For this review, take the finished solid that the model builds, in its own axes (mm). Face numbers are marked on the shaded views. A direction names the side the tool comes from. Round coordinates to 2 decimals unless told otherwise and drop trailing zeros. Write each loop counter-clockwise with the first axis right and the second up, starting at its lowest first coordinate (ties: lowest second). Pieces come first, ordered by that corner, then holes.
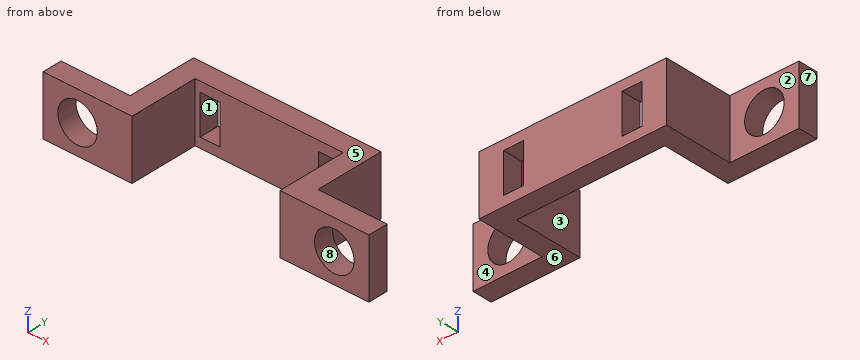
from build123d import *

# Parameters (mm, degrees)
CYLINDER001_R     = 2
CYLINDER001_DEPTH = 10
BOX004_W          = 7
BOX004_H          = 2
BOX004_DEPTH      = 6
BOX002_W          = 2
BOX002_H          = 7
BOX002_DEPTH      = 6
BOX001_W          = 2
BOX001_H          = 7
BOX001_DEPTH      = 6
CYLINDER_R        = 2
CYLINDER_DEPTH    = 10
BOX003_W          = 7
BOX003_H          = 2
BOX003_DEPTH      = 6
BOX006_W          = 2
BOX006_H          = 6
BOX006_DEPTH      = 4
BOX005_W          = 2
BOX005_H          = 6
BOX005_DEPTH      = 4
BOX_W             = 19
BOX_H             = 2
BOX_DEPTH         = 6


with BuildPart() as cylinder001:
    # Cylinder001 → Cylinder001 (new body)
    with BuildSketch(Plane(origin=(22.5, 0, 3), x_dir=(1, 0, 0), z_dir=(0, -1, 0))):
        Circle(CYLINDER001_R)
    extrude(amount=CYLINDER001_DEPTH)


with BuildPart() as cut001:
    # Box004 → Box004 (new body)
    with BuildSketch(Plane(origin=(19, -7, 0), x_dir=(1, 0, 0), z_dir=(0, 0, 1))):
        with Locations((3.5, 1)):
            Rectangle(BOX004_W, BOX004_H)
    extrude(amount=BOX004_DEPTH)

    # Cut001: cut Cylinder001
    add(cylinder001.part, mode=Mode.SUBTRACT)


with BuildPart() as cube002:
    # Box002 → Box002 (new body)
    with BuildSketch(Plane(origin=(17, -7, 0), x_dir=(1, 0, 0), z_dir=(0, 0, 1))):
        with Locations((1, 3.5)):
            Rectangle(BOX002_W, BOX002_H)
    extrude(amount=BOX002_DEPTH)


with BuildPart() as cube001:
    # Box001 → Box001 (new body)
    with BuildSketch(Plane(origin=(0, -7, 0), x_dir=(1, 0, 0), z_dir=(0, 0, 1))):
        with Locations((1, 3.5)):
            Rectangle(BOX001_W, BOX001_H)
    extrude(amount=BOX001_DEPTH)


with BuildPart() as cylinder:
    # Cylinder → Cylinder (new body)
    with BuildSketch(Plane(origin=(-3.5, 0, 3), x_dir=(1, 0, 0), z_dir=(0, -1, 0))):
        Circle(CYLINDER_R)
    extrude(amount=CYLINDER_DEPTH)


with BuildPart() as fusion:
    # Box003 → Box003 (new body)
    with BuildSketch(Plane(origin=(-7, -7, 0), x_dir=(1, 0, 0), z_dir=(0, 0, 1))):
        with Locations((3.5, 1)):
            Rectangle(BOX003_W, BOX003_H)
    extrude(amount=BOX003_DEPTH)

    # Cut: cut Cylinder
    add(cylinder.part, mode=Mode.SUBTRACT)

    # Fusion: union Cube001
    add(cube001.part)


with BuildPart() as cube006:
    # Box006 → Box006 (new body)
    with BuildSketch(Plane(origin=(14.5, -3, 1), x_dir=(1, 0, 0), z_dir=(0, 0, 1))):
        with Locations((1, 3)):
            Rectangle(BOX006_W, BOX006_H)
    extrude(amount=BOX006_DEPTH)


with BuildPart() as cube005:
    # Box005 → Box005 (new body)
    with BuildSketch(Plane(origin=(2.5, -3, 1), x_dir=(1, 0, 0), z_dir=(0, 0, 1))):
        with Locations((1, 3)):
            Rectangle(BOX005_W, BOX005_H)
    extrude(amount=BOX005_DEPTH)


with BuildPart() as fusion003:
    # Box → Box (new body)
    with BuildSketch(Plane.XY):
        with Locations((9.5, 1)):
            Rectangle(BOX_W, BOX_H)
    extrude(amount=BOX_DEPTH)

    # Cut002: cut Cube005
    add(cube005.part, mode=Mode.SUBTRACT)

    # Cut003: cut Cube006
    add(cube006.part, mode=Mode.SUBTRACT)

    # Fusion001: union Fusion
    add(fusion.part)

    # Fusion002: union Cube002
    add(cube002.part)

    # Fusion003: union Cut001
    add(cut001.part)


solid = fusion003.part
(1) For the marked faces 1, 2, 3 and 4, list the 3-axis set-ups (+Z, -Z, +X, -X, +Y, -Y) from which the entire face can be reached by the end or side of a thin tool; tool diameter is ignored.
Geometry check:
face 1: +Y, -Y
face 2: +Z, -Z, -X, +Y
face 3: +Z, -Z, -Y
face 4: +Z, -Z, +X, +Y
(2) Mouldability with a two-part tool opening along Z and no side actions: class the marked faces 5, 6, 7 and 8 as pulls with the +Z half, pulls with the -Z half, needs draft (parallel to the pull), parting line crosses it, or undercut.
Geometry check:
face 5: pulls with the +Z half
face 6: pulls with the -Z half
face 7: needs draft
face 8: undercut
(3) We need section B-B, the plane z = 3. Give the boundary of the cut face in (x, y), and give its area (3 significant figures).
Geometry check:
outline: (-7, -7) - (-5.5, -7) - (-5.5, -5) - (-7, -5) - close; (-1.5, -7) - (2, -7) - (2, 0) - (2.5, 0) - (2.5, 2) - (0, 2) - (0, -5) - (-1.5, -5) - close; (4.5, 0) - (14.5, 0) - (14.5, 2) - (4.5, 2) - close; (16.5, 0) - (17, 0) - (17, -7) - (20.5, -7) - (20.5, -5) - (19, -5) - (19, 2) - (16.5, 2) - close; (24.5, -7) - (26, -7) - (26, -5) - (24.5, -5) - close
area: 70.0 mm2
(4) We need section D-D, the plane y = -0.5. Give the boundary of the cut face in (x, z), and give its area (3 significant figures).
Geometry check:
outline: (0, 0) - (2, 0) - (2, 6) - (0, 6) - close; (17, 0) - (19, 0) - (19, 6) - (17, 6) - close
area: 24.0 mm2
(5) For pin 1 Ø3 at (x, z) = (22.5, 3) entering from +Y; pin 2 Ø0.6 at (y, z) = (1.5, 4) entering from +X; pin 3 Ø1.8 at (y, z) = (0, 3) entering from -X; pin 4 Ø3 at (x, z) = (8, 2) entering from -Y, all flat-tipped, find the tip position at first contact; note any pin that passes through.
Geometry check:
pin 1: passes through
pin 2: stops at x = 19
pin 3: stops at x = 0
pin 4: stops at y = 0
(6) We need section A-A, the plane y = -6.5. Give the boundary of the cut face in (x, z), and give its area (3 significant figures).
Geometry check:
outline: (-7, 0) - (2, 0) - (2, 6) - (-7, 6) - close; (17, 0) - (26, 0) - (26, 6) - (17, 6) - close; hole circle Ø4 at (-3.5, 3); hole circle Ø4 at (22.5, 3)
area: 82.9 mm2
(7) We need section C-C, the plane x = 22.5. Give the boundary of the cut face in (y, z).
Geometry check:
outline: (-7, 0) - (-5, 0) - (-5, 1) - (-7, 1) - close; (-7, 5) - (-5, 5) - (-5, 6) - (-7, 6) - close
(8) For line 1 along X through (y, z) = (-5.35, 3); line 2 along X through (y, z) = (-0.5, 0.85); line 3 along Z through (x, y) = (22.5, -6.1), list the stretches that pass through material, from the lowest coordinate up.
Geometry check:
line 1: x = -7 to -5.5, -1.5 to 2, 17 to 20.5, 24.5 to 26
line 2: x = 0 to 2, 17 to 19
line 3: z = 0 to 1, 5 to 6
